Geometry: see drawing. Coordinates: mm, zero at the bounding-box minimum. Coordinates: 2 decimals unless noted, no trailing zeros. Write each loop counter-clockwise with the first axis right and the second up, starting at its lowest first coordinate (ties: lowest second). Pieces come first, ordered by that corner, then holes.
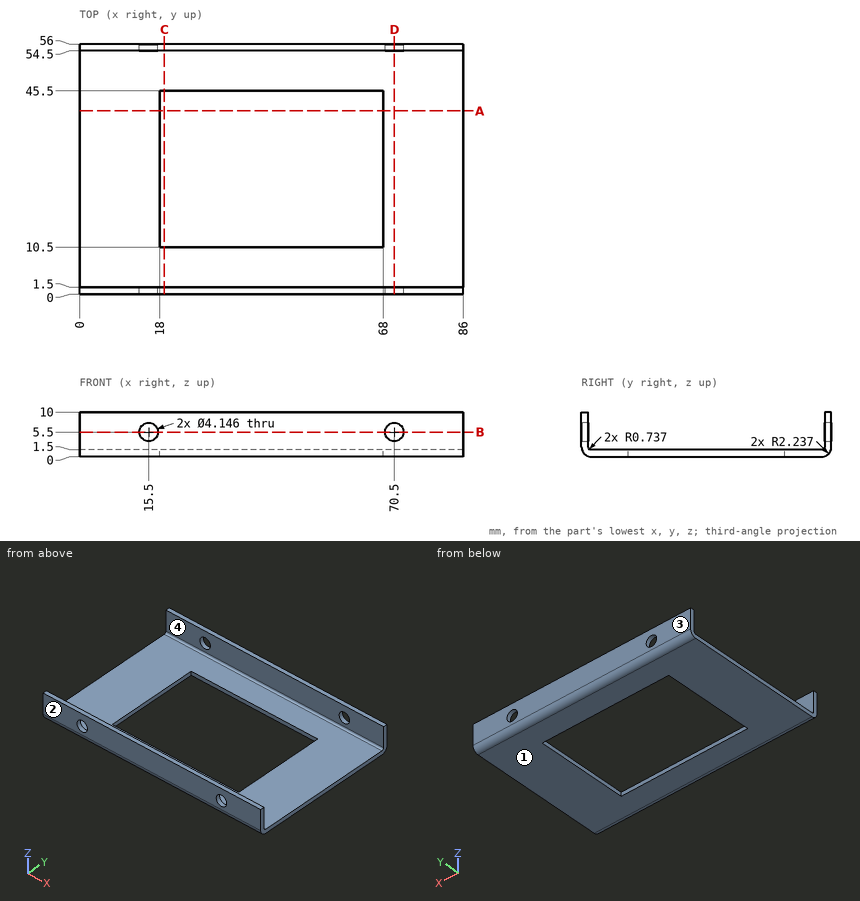
Item 1: Section D-D, the plane x = 70.5. Output: boundary loops of the cut face in (y, z).
Derived:
outline: (0, 2.24) arc R2.24 ccw to (2.24, 0) - (53.76, 0) arc R2.24 ccw to (56, 2.24) - (56, 3.43) - (54.5, 3.43) - (54.5, 2.24) arc R0.74 cw to (53.76, 1.5) - (2.24, 1.5) arc R0.74 cw to (1.5, 2.24) - (1.5, 3.43) - (0, 3.43) - close; (0, 7.57) - (1.5, 7.57) - (1.5, 10) - (0, 10) - close; (54.5, 7.57) - (56, 7.57) - (56, 10) - (54.5, 10) - close
Item 2: Pull-direction query (Y, two-part tool) for the marked faces 1, 2, 3 and 4; classes: released by +Y, released by -Y, zero draft, split by the parting line, or undercut.
Derived:
face 1: zero draft
face 2: released by -Y
face 3: released by +Y
face 4: undercut
Item 3: Section B-B, the plane z = 5.5. Output: boundary loops of the cut face in (x, y), plus the area to 3 significant figures.
Derived:
outline: (0, 0) - (13.43, 0) - (13.43, 1.5) - (0, 1.5) - close; (0, 54.5) - (13.43, 54.5) - (13.43, 56) - (0, 56) - close; (17.57, 0) - (68.43, 0) - (68.43, 1.5) - (17.57, 1.5) - close; (17.57, 54.5) - (68.43, 54.5) - (68.43, 56) - (17.57, 56) - close; (72.57, 0) - (86, 0) - (86, 1.5) - (72.57, 1.5) - close; (72.57, 54.5) - (86, 54.5) - (86, 56) - (72.57, 56) - close
area: 233 mm2
Item 4: Section C-C, the plane x = 19. Output: boundary loops of the cut face in (y, z).
Derived:
outline: (0, 2.24) arc R2.24 ccw to (2.24, 0) - (10.5, 0) - (10.5, 1.5) - (2.24, 1.5) arc R0.74 cw to (1.5, 2.24) - (1.5, 10) - (0, 10) - close; (45.5, 0) - (53.76, 0) arc R2.24 ccw to (56, 2.24) - (56, 10) - (54.5, 10) - (54.5, 2.24) arc R0.74 cw to (53.76, 1.5) - (45.5, 1.5) - close
Item 5: Material intervals for probe 1 along X at (y, z) = (0.8, 5.5); probe 2 along Y at (x, z) = (46, 9.5); probe 3 along X at (y, z) = (16.5, 1.25), sorted ascending.
Derived:
probe 1: x = 0 to 13.43, 17.57 to 68.43, 72.57 to 86
probe 2: y = 0 to 1.5, 54.5 to 56
probe 3: x = 0 to 18, 68 to 86
Item 6: Section A-A, the plane y = 41. Output: boundary loops of the cut face in (x, z).
Derived:
outline: (0, 0) - (18, 0) - (18, 1.5) - (0, 1.5) - close; (68, 0) - (86, 0) - (86, 1.5) - (68, 1.5) - close
Item 7: Pin query (flat end, axial travel): pin 1 (6 mm diameter, centred on y = 39.5, z = 4, fed in from +X); pin 2 (3.5 mm diameter, centred on x = 15.5, z = 5.5, fed in from +Y); pin 3 (1.5 mm diameter, centred on x = 23, z = 1, fed in from +Y); pin 4 (12 mm diameter, centred on x = 14.5, y = 19.5, fed in from +Z). Return the tip coordinate at first contact, or that it passes through.
Derived:
pin 1: stops at x = 86
pin 2: passes through
pin 3: stops at y = 55.95
pin 4: stops at z = 1.5
